```python
from build123d import *

# Parameters (mm, degrees)
SKETCH1_W           = 20
SKETCH1_H           = 20
BOSS_EXTRUDE1_DEPTH = 2.5
SKETCH2_R           = 1.1
CUT_EXTRUDE1_DEPTH  = 21
SKETCH3_R           = 2
CUT_EXTRUDE2_DEPTH  = 3.5


with BuildPart() as part:
    # Sketch1 → Boss-Extrude1 (new body)
    with BuildSketch(Plane(origin=(0, 0, 0), x_dir=(1, 0, 0), z_dir=(0, 1, 0))):
        with Locations((-50.754716981, 42.075471698)):
            Rectangle(SKETCH1_W, SKETCH1_H)
    extrude(amount=BOSS_EXTRUDE1_DEPTH)

    # Sketch2 → Cut-Extrude1 (cut, through all)
    with BuildSketch(Plane.XY.offset(-32.075471698)):
        with Locations((-50.754716981, 2.75)):
            Circle(SKETCH2_R)
    extrude(amount=-CUT_EXTRUDE1_DEPTH, mode=Mode.SUBTRACT)

    # Sketch3 → Cut-Extrude2 (cut, through all)
    with BuildSketch(Plane(origin=(0, 2.5, 0), x_dir=(1, 0, 0), z_dir=(0, 1, 0))):
        with Locations((-55.754716981, 42.075471698)):
            Circle(SKETCH3_R)
        with Locations((-45.754716981, 42.075471698)):
            Circle(SKETCH3_R)
    extrude(amount=-CUT_EXTRUDE2_DEPTH, mode=Mode.SUBTRACT)


solid = part.part
```
Check sheet for the modelled part. Datum: model origin and axes. Units: mm. Give positions to 0.01 mm unless a question says otherwise; leave off trailing zeros. Write each loop counter-clockwise with the first axis right and the second up, starting at its lowest first coordinate (ties: lowest second). Pieces come first, ordered by that corner, then holes.
Item 1: Cross-section at B-B (z = -41.25). Enter the section's corners in (x, y).
Item 2: Scan lines: L1, parallel to X at y = 0.55, z = -43; L2, parallel to Z at x = -55.5, y = 0.25; L3, parallel to X at y = 2.05, z = -36.5. Record each from-to range of solid material in increasing order.
Item 3: Draft check along X on faces 1 (the face through (-50.78, 1.65, -41.94)), 2 (the face through (-51, 0, -42)), 3 (the face through (-40.755, 1, -42)). Enter one of: released by +X, released by -X, zero draft, split by the parting line, or undercut.
Item 4: Cross-section at A-A (x = -55). Enter the section's corners in (y, z), and give its area (3 significant figures).
Item 5: Cross-section at C-C (y = 2.2). Enter the section's corners in (x, z).
Item 6: Cross-section at D-D (x = -45.5). Enter the section's corners in (y, z).
Report:
1. outline: (-60.75, 0) - (-57.58, 0) - (-57.58, 2.5) - (-60.75, 2.5) - close; (-53.93, 0) - (-47.58, 0) - (-47.58, 2.5) - (-49.68, 2.5) arc R1.1 cw to (-51.83, 2.5) - (-53.93, 2.5) - close; (-43.93, 0) - (-40.75, 0) - (-40.75, 2.5) - (-43.93, 2.5) - close
2. L1: x = -60.75 to -57.53, -53.98 to -47.53, -43.98 to -40.75
2. L2: z = -52.08 to -44.06, -40.09 to -32.08
2. L3: x = -60.75 to -51.6, -49.91 to -40.75
3. face 1: undercut
3. face 2: zero draft
3. face 3: released by +X
4. outline: (0, -52.08) - (2.5, -52.08) - (2.5, -43.93) - (0, -43.93) - close; (0, -40.22) - (2.5, -40.22) - (2.5, -32.08) - (0, -32.08) - close
4. area: 40.7 mm2
5. outline: (-60.75, -52.08) - (-51.71, -52.08) - (-51.71, -32.08) - (-60.75, -32.08) - close; (-49.8, -52.08) - (-40.75, -52.08) - (-40.75, -32.08) - (-49.8, -32.08) - close; hole circle Ø4 at (-55.75, -42.08); hole circle Ø4 at (-45.75, -42.08)
6. outline: (0, -52.08) - (2.5, -52.08) - (2.5, -44.06) - (0, -44.06) - close; (0, -40.09) - (2.5, -40.09) - (2.5, -32.08) - (0, -32.08) - close
